```python
from build123d import *

# Parameters (mm, degrees)
CROQUIS1_W                                           = 47
CROQUIS1_H                                           = 49
SALIENTE_EXTRUIR1_DEPTH                              = 3
CROQUIS14_W                                          = 7
CROQUIS14_H                                          = 7
SALIENTE_EXTRUIR4_DEPTH                              = 8
TALADRO_DE_MARGEN_PARA_M35_D                         = 3.2
REFRENTADO_PARA_TORNILLO_CON_CABEZA_PLAN_D           = 3.4
REFRENTADO_PARA_TORNILLO_CON_CABEZA_PLAN_CBORE_D     = 6.5
REFRENTADO_PARA_TORNILLO_CON_CABEZA_PLAN_CBORE_DEPTH = 2
CROQUIS25_R                                          = 4.75
CORTAR_EXTRUIR4_DEPTH                                = 2.54


with BuildPart() as part:
    # Croquis1 → Saliente-Extruir1 (new body)
    with BuildSketch(Plane(origin=(0, 0, 0), x_dir=(1, 0, 0), z_dir=(0, 1, 0))):
        with Locations((23.5, 24.5)):
            Rectangle(CROQUIS1_W, CROQUIS1_H)
    extrude(amount=SALIENTE_EXTRUIR1_DEPTH)

    # Croquis14 → Saliente-Extruir4 (add)
    with BuildSketch(Plane(origin=(0, 3, 0), x_dir=(1, 0, 0), z_dir=(0, 1, 0))):
        with Locations((3.5, 45.5)):
            Rectangle(CROQUIS14_W, CROQUIS14_H)
        with Locations((43.5, 45.5)):
            Rectangle(CROQUIS14_W, CROQUIS14_H)
        with Locations((43.5, 3.5)):
            Rectangle(CROQUIS14_W, CROQUIS14_H)
        with Locations((3.5, 3.5)):
            Rectangle(CROQUIS14_W, CROQUIS14_H)
    extrude(amount=SALIENTE_EXTRUIR4_DEPTH)

    # Taladro de margen para M35 (through all)
    with Locations(Plane(origin=(3, 0, -4), x_dir=(0, 0, -1), z_dir=(0, -1, 0))):
        with Locations((0, 0), (0, 41), (41, 41), (41, 0)):
            Hole(TALADRO_DE_MARGEN_PARA_M35_D / 2)

    # Refrentado para tornillo con cabeza plana de M31 (through all)
    with Locations(Plane(origin=(22.5, 0, -7), x_dir=(0, 0, -1), z_dir=(0, -1, 0))):
        with Locations((0, 0), (35, 0)):
            CounterBoreHole(REFRENTADO_PARA_TORNILLO_CON_CABEZA_PLAN_D / 2, REFRENTADO_PARA_TORNILLO_CON_CABEZA_PLAN_CBORE_D / 2, REFRENTADO_PARA_TORNILLO_CON_CABEZA_PLAN_CBORE_DEPTH)

    # Croquis25 → Cortar-Extruir4 (cut)
    with BuildSketch(Plane.XZ):
        with Locations(Location((11.75, -12.25, 0), (0, 0, 270))):
            Circle(CROQUIS25_R)
        with Locations(Location((35.25, -12.25, 0), (0, 0, 90))):
            Circle(CROQUIS25_R)
        with Locations(Location((35.25, -36.75, 0), (0, 0, 270))):
            Circle(CROQUIS25_R)
        with Locations(Location((11.75, -36.75, 0), (0, 0, 90))):
            Circle(CROQUIS25_R)
    extrude(amount=-CORTAR_EXTRUIR4_DEPTH, mode=Mode.SUBTRACT)


solid = part.part
```
Model file for the job. Use its own axes, mm. A direction names the side the tool comes from. Round coordinates to 2 decimals unless told otherwise and drop trailing zeros. Loops run counter-clockwise (first coordinate to the right, second up) from the corner with the lowest first, then second, coordinate; pieces in that order, holes last. Notation, with made-up numbers: M -23,31.25 L 12,31.25 A30 ccw 12,59.25 Z; hole C -0.75,46 d1. An arc over 180 degrees is marked long. Put each result on its own line as item: value. Start each with the question number.
Item 1: Cut at B-B (x = 44). List the corners of the cut face in (y, z).
Item 2: Drill centre lines: line 1 along X through (y, z) = (0.85, -12.25); line 2 along X through (y, z) = (0.7, -42); line 3 along Z through (x, y) = (4, 3.25). Where is each one in solid material? Low to high.
Item 3: 3-axis set-ups, long thin cutter, end or side, ignore diameter. For faces 3 (the face through (47, 2, -24)), 4 (the face through (12, 2.54, -12)), 5 (the face through (42.7, 11, -2.8)), 6 (the face through (3, 7, -7)), 7 (the face through (40, 7, -45)): which of +Z, -Z, +X, -X, +Y, -Y reach the whole face in a straight line?
Item 4: Cut at A-A (y = 9). List the corners of the cut face in (x, z).
Item 5: Cut at D-D (z = -12.25). List the corners of the cut face in (x, y), then the cut area to 3 significant figures.
Item 6: Cut at C-C (x = 11.75). List the corners of the cut face in (y, z), then the cut area to 3 significant figures.
Item 7: Mould opens along Z. For faces 1 (the face through (23, 0, -25)), 2 (the face through (21.1, 2, -8.4)) say: released by +Z, released by -Z, zero draft, split by the parting line, or undercut.
Item 8: Drop flat-ended pins along their axis: P1, Ø12, axis at x = 28.5, z = -26, coming from the +Y side; P2, Ø5, axis at x = 34.5, z = -36.5, coming from the -Y side. Give the stop position or say it passes through.
Answer block:
1. outline: M 0,-49 L 11,-49 L 11,-46.6 L 0,-46.6 Z; M 0,-43.4 L 11,-43.4 L 11,-42 L 3,-42 L 3,-7 L 11,-7 L 11,-5.6 L 0,-5.6 Z; M 0,-2.4 L 11,-2.4 L 11,0 L 0,0 Z
2. line 1: 0 to 7, 16.5 to 30.5, 40 to 47
2. line 2: 0 to 19.25, 25.75 to 47
2. line 3: -49 to -46.25, -43.75 to -42, -7 to -5.25, -2.75 to 0
3. face 3: +Z, -Z, +X, +Y, -Y
3. face 4: -Y
3. face 5: +Z, -Z, +X, -X, +Y
3. face 6: +X, -X, +Y
3. face 7: +Z, -Z, +Y
4. outline: M 0,-49 L 7,-49 L 7,-42 L 0,-42 Z; M 0,-7 L 7,-7 L 7,0 L 0,0 Z; M 40,-49 L 47,-49 L 47,-42 L 40,-42 Z; M 40,-7 L 47,-7 L 47,0 L 40,0 Z; hole C 3,-45 d3.2; hole C 3,-4 d3.2; hole C 44,-45 d3.2; hole C 44,-4 d3.2
5. outline: M 0,0 L 7,0 L 7,2.54 L 16.5,2.54 L 16.5,0 L 30.5,0 L 30.5,2.54 L 40,2.54 L 40,0 L 47,0 L 47,3 L 0,3 Z
5. area: 92.7 mm2
6. outline: M 0,-49 L 3,-49 L 3,0 L 0,0 L 0,-7.5 L 2.54,-7.5 L 2.54,-17 L 0,-17 L 0,-32 L 2.54,-32 L 2.54,-41.5 L 0,-41.5 Z
6. area: 98.7 mm2
7. face 1: zero draft
7. face 2: undercut
8. P1: y = 3
8. P2: y = 2.54
